For this review, take the finished solid that the model builds, in its own axes (mm). Round coordinates to 2 decimals unless told otherwise and drop trailing zeros. Write each loop counter-clockwise with the first axis right and the second up, starting at its lowest first coordinate (ties: lowest second). Pieces come first, ordered by that corner, then holes.
from build123d import *

# Parameters (mm, degrees)
SKETCH_1_W      = 45
SKETCH_1_H      = 20
SKETCH_1_R      = 2.1
EXTRUDE_1_DEPTH = 3
FILLET_1_R      = 3


with BuildPart() as part:
    # 草图1 → 凸台-拉伸1 (new body)
    with BuildSketch(Plane(origin=(0, 0, 0), x_dir=(1, 0, 0), z_dir=(0, 1, 0))):
        with Locations((12.5, 0)):
            Rectangle(SKETCH_1_W, SKETCH_1_H)
        with Locations(Location((0, 0, 0), (0, 0, 270))):
            Circle(SKETCH_1_R, mode=Mode.SUBTRACT)
        with Locations(Location((25, 0, 0), (0, 0, 270))):
            Circle(SKETCH_1_R, mode=Mode.SUBTRACT)
    extrude(amount=EXTRUDE_1_DEPTH)

    # 圆角1
    fillet_1_edges = [part.edges().sort_by_distance(p)[0] for p in [
        (35, 1.5, 10),
        (-10, 1.5, 10),
        (-10, 1.5, -10),
        (35, 1.5, -10),
    ]]
    fillet(fillet_1_edges, radius=FILLET_1_R)


solid = part.part
(1) Mouldability with a two-part tool opening along X and no side actions: class faces 1 (the face through (34.1, 1.52, 9.14)), 2 (the face through (12, 1, -10)), 3 (the face through (26.77, 1.48, 1.13)) as pulls with the +X half, pulls with the -X half, needs draft (parallel to the pull), parting line crosses it, or undercut.
Geometry check:
face 1: pulls with the +X half
face 2: needs draft
face 3: undercut
(2) We need section C-C, the plane y = 2.2. Give the boundary of the cut face in (x, z).
Geometry check:
outline: (-10, -7) arc R3 ccw to (-7, -10) - (32, -10) arc R3 ccw to (35, -7) - (35, 7) arc R3 ccw to (32, 10) - (-7, 10) arc R3 ccw to (-10, 7) - close; hole circle Ø4.2 at (0, 0); hole circle Ø4.2 at (25, 0)
(3) We need section A-A, the plane x = 0. Give the boundary of the cut face in (y, z), and give its area (3 significant figures).
Geometry check:
outline: (0, -10) - (3, -10) - (3, -2.1) - (0, -2.1) - close; (0, 2.1) - (3, 2.1) - (3, 10) - (0, 10) - close
area: 47.4 mm2
(4) For line 1 along X through (y, z) = (1.5, 0); line 2 along X through (y, z) = (2.4, -1.25); line 3 along X through (y, z) = (2.6, 7.25), list the stretches that pass through material, from the lowest coordinate up.
Geometry check:
line 1: x = -10 to -2.1, 2.1 to 22.9, 27.1 to 35
line 2: x = -10 to -1.69, 1.69 to 23.31, 26.69 to 35
line 3: x = -9.99 to 34.99
(5) We need section B-B, the plane z = 0. Give the boundary of the cut face in (x, y).
Geometry check:
outline: (-10, 0) - (-2.1, 0) - (-2.1, 3) - (-10, 3) - close; (2.1, 0) - (22.9, 0) - (22.9, 3) - (2.1, 3) - close; (27.1, 0) - (35, 0) - (35, 3) - (27.1, 3) - close
(6) For pin 1 Ø3.5 at (x, z) = (0, 0) entering from -Y, flat-tipped, find the tip position at first contact; note if it passes through.
Geometry check:
pin 1: passes through
(7) We need section D-D, the plane x = 26.5. Give the boundary of the cut face in (y, z), and give its area (3 significant figures).
Geometry check:
outline: (0, -10) - (3, -10) - (3, -1.47) - (0, -1.47) - close; (0, 1.47) - (3, 1.47) - (3, 10) - (0, 10) - close
area: 51.2 mm2
